Model file for the job. Use its own axes, mm. Coordinates: 2 decimals unless noted, no trailing zeros. Write each loop counter-clockwise with the first axis right and the second up, starting at its lowest first coordinate (ties: lowest second). Pieces come first, ordered by that corner, then holes. Notation, with made-up numbers: (-17, 4) - (-3, 4) arc R22 ccw to (-3, 27) - close; hole circle Ø3 at (75.5, 60). An arc over 180 degrees is marked (long way). Put each result on its own line as item: value. Start each with the question number.
1. Saw through at A-A, the plane x = 18.5. Write the cut outline in (y, z), plus the area to 3 significant figures.
2. Saw through at B-B, the plane z = 0. Write the cut outline in (x, y).
3. Saw through at C-C, the plane y = -0.85. Write the cut outline in (x, z).
4. Saw through at D-D, the plane x = 0. Write the cut outline in (y, z).
5. Drill centre lines: L1, parallel to Z at x = 0, y = -0.6; L2, parallel to X at y = -0.6, z = 21.5; L3, parallel to Z at x = -1, y = -0.75. Where is each one in solid material? Low to high. Write a range as from..to.
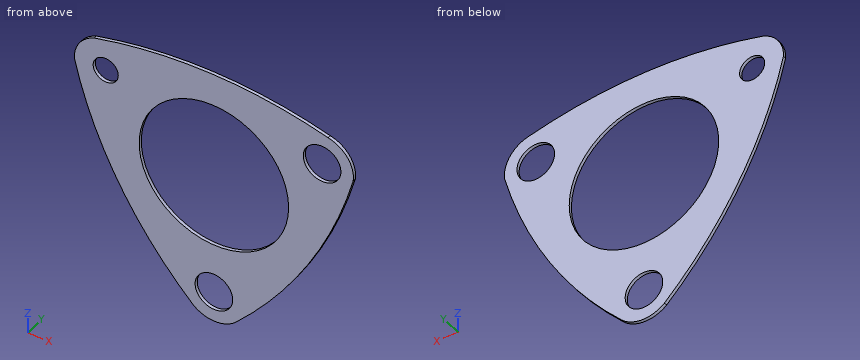
```python
from build123d import *

# Parameters (mm, degrees)
F0_R     = 6
F0_R_2   = 4
F0_R_3   = 23.837169
F1_DEPTH = 1


with BuildPart() as f1:
    # F0 (on Front) → F1 (new body)
    with BuildSketch(Plane.XZ):
        with BuildLine():
            ThreePointArc((36.439317, 29.728735), (-0.919317, 34.356199), (-38.209367, 29.205166))
            ThreePointArc((-38.209367, 29.205166), (-42.945645, 25.273123), (-44.48159, 19.312069))
            ThreePointArc((-44.48159, 19.312069), (-30.280128, -16.75426), (-6.54421, -47.398472))
            ThreePointArc((-6.54421, -47.398472), (0.429493, -49.827941), (7.168973, -46.808956))
            ThreePointArc((7.168973, -46.808956), (30.038151, -16.547447), (44.406826, 18.556677))
            ThreePointArc((44.406826, 18.556677), (42.641652, 25.724917), (36.439317, 29.728735))
        make_face()
        with Locations((0, -39.837169)):
            Circle(F0_R, mode=Mode.SUBTRACT)
        with Locations((-34.5, 19.918584)):
            Circle(F0_R_2, mode=Mode.SUBTRACT)
        Circle(F0_R_3, mode=Mode.SUBTRACT)
        with Locations((34.5, 19.918584)):
            Circle(F0_R, mode=Mode.SUBTRACT)
    extrude(amount=F1_DEPTH)


solid = f1.part
```
Final values:
1. outline: (-1, -33.83) - (0, -33.83) - (0, -15.03) - (-1, -15.03) - close; (-1, 15.03) - (0, 15.03) - (0, 33.19) - (-1, 33.19) - close
1. area: 37.0 mm²
2. outline: (-38.36, -1) - (-23.84, -1) - (-23.84, 0) - (-38.36, 0) - close; (23.84, -1) - (38.14, -1) - (38.14, 0) - (23.84, 0) - close
3. outline: (-44.48, 19.31) arc R136.98 ccw to (-6.54, -47.4) arc R10 ccw to (7.17, -46.81) arc R147.07 ccw to (44.41, 18.56) arc R10 ccw to (36.44, 29.73) arc R144.91 ccw to (-38.21, 29.21) arc R10 ccw to start; hole circle Ø8 at (-34.5, 19.92); hole circle Ø47.67 at (0, 0); hole circle Ø12 at (0, -39.84); hole circle Ø12 at (34.5, 19.92)
4. outline: (-1, -49.84) - (0, -49.84) - (0, -45.84) - (-1, -45.84) - close; (-1, -33.84) - (0, -33.84) - (0, -23.84) - (-1, -23.84) - close; (-1, 23.84) - (0, 23.84) - (0, 34.36) - (-1, 34.36) - close
5. L1: z = -49.84..-45.84, -33.84..-23.84, 23.84..34.36
5. L2: x = -44.37..-38.17, -30.83..-10.29, 10.29..28.71, 40.29..44.37
5. L3: z = -49.79..-45.75, -33.92..-23.82, 23.82..34.36
